Autodesk Inventor part; units mm, degrees
ref_plane "YZ Plane" through (0, 0, 0) normal (1, 0, 0) x (0, 1, 0)
ref_plane "XZ Plane" through (0, 0, 0) normal (0, 1, 0) x (-1, 0, 0)
ref_plane "XY Plane" through (0, 0, 0) normal (0, 0, 1) x (1, 0, 0)
sketch "Sketch1" plane through (0, 0, 0) normal (0, 1, 0) x (-1, 0, 0)
  circle A0 centre (0, 0) radius 3.4925
  circle A1 centre (24.13, 0) radius 3.4925
  line L0 (0, 1.4605) -> (24.13, 1.4605)
  line L1 (24.13, 1.4605) -> (24.13, -1.4605)
  line L2 (24.13, -1.4605) -> (0, -1.4605)
  line L3 (0, -1.4605) -> (0, 1.4605)
  dimension "d0" = 6.985
  dimension "d1" = 2.921
  dimension "d2" = 1.4605
  dimension "d3" = 24.13
  dimension "d4" = 6.985
extrude "Extrusion1" add sketch "Sketch1" along normal mid plane 5.08 contours A0 L2 L3 L0 | L0 L3 L2 A0 | L0 L1 L2 A1 | A1 L2 L1 L0
sketch "Sketch2" plane through (0, 0, 0) normal (0, 1, 0) x (-1, 0, 0)
  circle A0 centre (0, 0) radius 3.4925
  circle A1 centre (24.13, 0) radius 3.4925
  line L0 (0, 1.4605) -> (24.13, 1.4605)
  line L1 (24.13, 1.4605) -> (24.13, -1.4605)
  line L2 (24.13, -1.4605) -> (0, -1.4605)
  line L3 (0, -1.4605) -> (0, 1.4605)
  dimension "d7" = 6.985
  dimension "d8" = 2.921
  dimension "d9" = 1.4605
  dimension "d10" = 24.13
  dimension "d11" = 6.985
extrude "Extrusion2" add sketch "Sketch2" along normal mid plane 2.54 contours A0 L2 L3 L0 | A0 L0 A1 L2 | L0 L1 L2 A1 picked at (1.1642, 0) picked at (22.9658, 0)
hole "Hole1" at (-24.13, 2.54, 0) direction (0, -1, 0) diameter 3.4798 end through all
hole "Hole3" at (0, 2.54, 0) direction (0, -1, 0) diameter 3.4798 end through all
equation "\"d0\" = d4"
equation "\"d2\" = 0.5 * d1"
equation "\"d7\" = d11"
equation "\"d9\" = 0.5 * d8"
properties part number "Crankarm"
Source: CAD feature listing. Evaluate the final solid. Frame: model axes, mm. A direction names the side the tool comes from. Coordinates: 2 decimals unless noted, no trailing zeros. Loops run counter-clockwise (first coordinate to the right, second up) from the corner with the lowest first, then second, coordinate; pieces in that order, holes last. Notation, with made-up numbers: (71, 28.25) -> (92, 28.25) arc R10 cw to (92, 44.25) -> close; hole circle Ø2 at (-12.5, 86). An arc over 180 degrees is marked (long way). Answer in a Markdown table with one row per item. Add a question column.
Q1. Section D-D on z = 2. Return the cut outline in (x, y), and give its area (3 significant figures).
Q2. Reachability of faces 1 (the face through (-12, 0, 1.46)), 2 (the face through (1.06, -0.04, -1.38)) from +Z, -Z, +X, -X, +Y, -Y: full face, straight path, thin tool, end or side. Return the list, or none.
Q3. Section A-A on z = 0. Return the cut outline in (x, y), and give its area (3 significant figures).
Q4. Pull-direction query (X, two-part tool) for faces 3 (the face through (-25, 2.54, 2)), 4 (the face through (-12, 0, -1.46)); classes: pulls with the +X half, pulls with the -X half, needs draft (parallel to the pull), parting line crosses it, or undercut.
Q5. Section B-B on x = 0. Return the cut outline in (y, z).
Q6. Ray query, line 1 along X through (y, z) = (-1.5, 0); line 2 along X through (y, z) = (-0.75, 0); line 3 along Z through (x, y) = (0, -0.9). Return the intervals inside material, ascending.
Q7. Section C-C on y = 0.9. Return the cut outline in (x, z) (1 decimal).
Q8. Contact query for flat-ended pins moving along their axis: pin 1 Ø0.8 at (x, y) = (-9.5, -0.5) entering from +Z; pin 2 Ø2 at (x, y) = (-10, -0.5) entering from -Z; pin 3 Ø1.5 at (x, z) = (-16.5, 1.5) entering from -Y. Output: stop coordinate, or through.
Computed values:
| question | item | result |
|---|---|---|
| 1 | outline | (-26.99, -2.54) -> (-21.27, -2.54) -> (-21.27, 2.54) -> (-26.99, 2.54) -> close; (-2.86, -2.54) -> (2.86, -2.54) -> (2.86, 2.54) -> (-2.86, 2.54) -> close |
| 1 | area | 58.2 mm^2 |
| 2 | face 1 | +Z, +Y, -Y |
| 2 | face 2 | +Y, -Y |
| 3 | outline | (-27.62, -2.54) -> (-25.87, -2.54) -> (-25.87, 2.54) -> (-27.62, 2.54) -> close; (-22.39, -2.54) -> (-20.64, -2.54) -> (-20.64, -1.27) -> (-3.49, -1.27) -> (-3.49, -2.54) -> (-1.74, -2.54) -> (-1.74, 2.54) -> (-3.49, 2.54) -> (-3.49, 1.27) -> (-20.64, 1.27) -> (-20.64, 2.54) -> (-22.39, 2.54) -> close; (1.74, -2.54) -> (3.49, -2.54) -> (3.49, 2.54) -> (1.74, 2.54) -> close |
| 3 | area | 79.2 mm^2 |
| 4 | face 3 | needs draft |
| 4 | face 4 | undercut |
| 5 | outline | (-2.54, -3.49) -> (2.54, -3.49) -> (2.54, -1.74) -> (-2.54, -1.74) -> close; (-2.54, 1.74) -> (2.54, 1.74) -> (2.54, 3.49) -> (-2.54, 3.49) -> close |
| 6 | line 1 | x = -27.62 to -25.87, -22.39 to -20.64, -3.49 to -1.74, 1.74 to 3.49 |
| 6 | line 2 | x = -27.62 to -25.87, -22.39 to -1.74, 1.74 to 3.49 |
| 6 | line 3 | z = -3.49 to -1.74, 1.74 to 3.49 |
| 7 | outline | (-21, -1.5) -> (-3.2, -1.5) arc R3.5 ccw (long way) to (-3.2, 1.5) -> (-21, 1.5) arc R3.5 ccw (long way) to start; hole circle Ø3.5 at (-24.1, 0); hole circle Ø3.5 at (0, 0) |
| 8 | pin 1 | stops at z = 1.46 |
| 8 | pin 2 | stops at z = -1.46 |
| 8 | pin 3 | stops at y = -1.27 |
